Check sheet for the modelled part. Datum: model origin and axes. Units: mm. A direction names the side the tool comes from. Coordinates: 2 decimals unless noted, no trailing zeros. Loops run counter-clockwise (first coordinate to the right, second up) from the corner with the lowest first, then second, coordinate; pieces in that order, holes last.
```python
from build123d import *

# Parameters (mm, degrees)
F0_W     = 27.94
F0_H     = 12.7
F1_DEPTH = 27.94
F2_W     = 19.05
F2_H     = 6.35
F3_DEPTH = 25.4
F4_R     = 9.52499
F5_R     = 3.302
F6_DEPTH = 6.35
F7_W     = 1.5875
F7_H     = 12.7
F8_DEPTH = 22.225


# Not quite as in the source:
# - a fillet or chamfer is up to 0.001 mm smaller than in the source, because OpenCascade refuses the exact size


with BuildPart() as f1:
    # F0 (on Front) → F1 (new body)
    with BuildSketch(Plane.XZ):
        with Locations((-13.97, -199.4363271219)):
            Rectangle(F0_W, F0_H)
    extrude(amount=-F1_DEPTH)

    # F2 (on face) → F3 (join)
    with BuildSketch(Plane.XY.offset(-193.0863271219)):
        with Locations((-13.97, 13.97)):
            Rectangle(F2_W, F2_H)
    extrude(amount=F3_DEPTH)

    # F4 (radius 9.525 in the source; OpenCascade refuses exactly that, so slightly less here)
    f4_edges = [f1.edges().sort_by_distance(p)[0] for p in [
        (-4.445, 13.97, -167.686327),
        (-23.495, 13.97, -167.686327),
    ]]
    fillet(f4_edges, radius=F4_R)

    # F5 (on face) → F6 (cut)
    with BuildSketch(Plane.XZ.offset(-10.795)):
        with Locations((-13.97, -177.2113271219)):
            Circle(F5_R)
    extrude(amount=-F6_DEPTH, mode=Mode.SUBTRACT)

    # F7 (on face) → F8 (cut)
    with BuildSketch(Plane(origin=(-27.94, 0, 0), x_dir=(0, -1, 0), z_dir=(-1, 0, 0))):
        with Locations((-25.55875, -177.2113271219)):
            Rectangle(F7_W, F7_H)
    extrude(amount=-F8_DEPTH, mode=Mode.SUBTRACT)


solid = f1.part
```
1) Scan lines: line 1 (Z direction, x = -13.97, y = 13.75); line 2 (Z direction, x = -7.5, y = 17.75); line 3 (X direction, y = 13.75, z = -191) (3 decimals). Record each from-to range of solid material in increasing order.
Answer sheet:
line 1: z = -205.79 to -180.51, -173.91 to -167.69
line 2: z = -205.79 to -193.09
line 3: x = -23.495 to -4.445
2) Mould release check, pull along X, two halves, no side actions. Record for faces 1 (the cylindrical face through (-14.686, 13.926, -180.435)), 2 (the flat face through (0, 14, -200)), 3 (the flat face through (-14, 17.145, -181)): +X half, -X half, draft (parallel to the pull), parting line (faces both ways), or undercut.
Answer sheet:
face 1: undercut
face 2: +X half
face 3: draft
3) Section check B-B on x = -15.25. Enter the section's corners in (y, z) (3 decimals), plus the area to 3 significant figures.
Answer sheet:
outline: (0, -205.786) - (27.94, -205.786) - (27.94, -193.086) - (17.145, -193.086) - (17.145, -180.255) - (10.795, -180.255) - (10.795, -193.086) - (0, -193.086) - close; (10.795, -174.168) - (17.145, -174.168) - (17.145, -167.773) - (10.795, -167.773) - close
area: 477 mm2
4) Set-up check for faces 4 (the flat face through (-14, 0, -199)), 5 (the flat face through (-4.445, 14, -185)), 6 (the flat face through (-14, 14, -205.786)), 7 (the flat face through (-14, 10.795, -181)), 8 (the flat face through (-23.495, 14, -185)): record each of +Z, -Z, +X, -X, +Y, -Y from which the full face is reachable in a straight line by a thin tool's end or side.
Answer sheet:
face 4: +Z, -Z, +X, -X, -Y
face 5: +Z, +X, +Y, -Y
face 6: -Z, +X, -X, +Y, -Y
face 7: +Z, +X, -X, -Y
face 8: +Z, -X, +Y, -Y
5) Section check A-A on z = -176. Enter the section's corners in (x, y) (3 decimals).
Answer sheet:
outline: (-23.418, 10.795) - (-17.042, 10.795) - (-17.042, 17.145) - (-23.418, 17.145) - close; (-10.898, 10.795) - (-4.522, 10.795) - (-4.522, 17.145) - (-10.898, 17.145) - close
6) Depth check by flat-ended pin: pin 1 (1.5 mm diameter, centred on x = -8, y = 16.5, fed in from +Z); pin 2 (3 mm diameter, centred on y = 15.5, z = -185, fed in from -X) (3 decimals); pin 3 (15 mm diameter, centred on x = -15.5, z = -175.5, fed in from -Y) (3 decimals); pin 4 (5.5 mm diameter, centred on x = -13.97, z = -177.21, fed in from -Y). Enter the tip coordinate at first touch or a pass-through.
Answer sheet:
pin 1: stops at z = -169.24
pin 2: stops at x = -23.495
pin 3: stops at y = 10.795
pin 4: passes through
7) Section check D-D on y = 4. Enter the section's corners in (x, z), plus the area to 3 significant figures.
Answer sheet:
outline: (-27.94, -205.79) - (0, -205.79) - (0, -193.09) - (-27.94, -193.09) - close
area: 355 mm2
